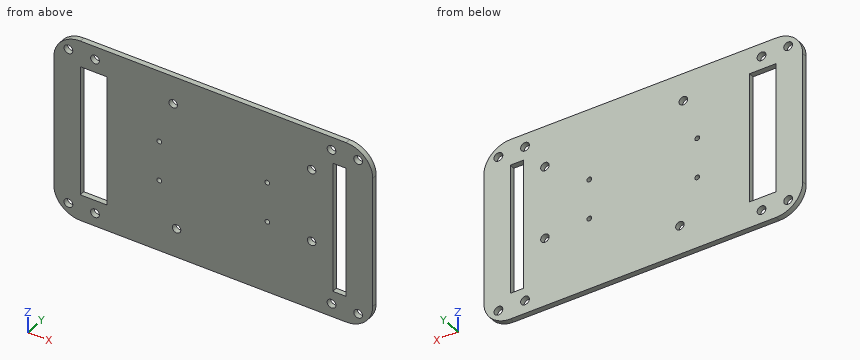
```python
from build123d import *

# Parameters (mm, degrees)
PLANTAICEZUM_W          = 120
PLANTAICEZUM_H          = 70
PLANTAICEZUM_R          = 1.6
SALIENTE_EXTRUIR3_DEPTH = 2
REDONDEO1_R             = 10
REDONDEO2_R             = 10
REDONDEO3_R             = 10
REDONDEO4_R             = 10
CROQUIS1_W              = 10
CROQUIS1_H              = 50
CROQUIS1_W_2            = 5
CORTAR_EXTRUIR1_DEPTH   = 5
CROQUIS4_R              = 1.65
CORTAR_EXTRUIR2_DEPTH   = 5
CROQUIS6_R              = 0.9
CORTAR_EXTRUIR4_DEPTH   = 10


with BuildPart() as part:
    # PlantaIceZum → Saliente-Extruir3 (new body)
    with BuildSketch(Plane(origin=(0, 0, 0), x_dir=(1, 0, 0), z_dir=(0, 1, 0))):
        with Locations((60, 35)):
            Rectangle(PLANTAICEZUM_W, PLANTAICEZUM_H)
        with Locations(Location((97, 43.66, 0), (0, 0, 270))):
            Circle(PLANTAICEZUM_R, mode=Mode.SUBTRACT)
        with Locations(Location((46.2, 58.9, 0), (0, 0, 270))):
            Circle(PLANTAICEZUM_R, mode=Mode.SUBTRACT)
        with Locations(Location((44.93, 10.64, 0), (0, 0, 270))):
            Circle(PLANTAICEZUM_R, mode=Mode.SUBTRACT)
        with Locations(Location((97, 15.72, 0), (0, 0, 270))):
            Circle(PLANTAICEZUM_R, mode=Mode.SUBTRACT)
    extrude(amount=SALIENTE_EXTRUIR3_DEPTH)

    # Redondeo1
    redondeo1_edges = [part.edges().sort_by_distance(p)[0] for p in [
        (0, 1, 0),
    ]]
    fillet(redondeo1_edges, radius=REDONDEO1_R)

    # Redondeo2
    redondeo2_edges = [part.edges().sort_by_distance(p)[0] for p in [
        (0, 1, -70),
    ]]
    fillet(redondeo2_edges, radius=REDONDEO2_R)

    # Redondeo3
    redondeo3_edges = [part.edges().sort_by_distance(p)[0] for p in [
        (120, 1, -70),
    ]]
    fillet(redondeo3_edges, radius=REDONDEO3_R)

    # Redondeo4
    redondeo4_edges = [part.edges().sort_by_distance(p)[0] for p in [
        (120, 1, 0),
    ]]
    fillet(redondeo4_edges, radius=REDONDEO4_R)

    # Croquis1 → Cortar-Extruir1 (cut)
    with BuildSketch(Plane(origin=(0, 2, 0), x_dir=(1, 0, 0), z_dir=(0, 1, 0))):
        with Locations((15, 35)):
            Rectangle(CROQUIS1_W, CROQUIS1_H)
        with Locations((107.5, 35)):
            Rectangle(CROQUIS1_W_2, CROQUIS1_H)
    extrude(amount=-CORTAR_EXTRUIR1_DEPTH, mode=Mode.SUBTRACT)

    # Croquis4 → Cortar-Extruir2 (cut)
    with BuildSketch(Plane(origin=(0, 2, 0), x_dir=(1, 0, 0), z_dir=(0, 1, 0))):
        with Locations(Location((5.5, 65, 0), (0, 0, 270))):
            Circle(CROQUIS4_R)
        with Locations(Location((114.5, 65, 0), (0, 0, 270))):
            Circle(CROQUIS4_R)
        with Locations(Location((5.5, 5, 0), (0, 0, 270))):
            Circle(CROQUIS4_R)
        with Locations(Location((114.5, 5, 0), (0, 0, 270))):
            Circle(CROQUIS4_R)
        with Locations(Location((15.5, 65, 0), (0, 0, 270))):
            Circle(CROQUIS4_R)
        with Locations(Location((104.5, 65, 0), (0, 0, 270))):
            Circle(CROQUIS4_R)
        with Locations(Location((15.5, 5, 0), (0, 0, 270))):
            Circle(CROQUIS4_R)
        with Locations(Location((104.5, 5, 0), (0, 0, 270))):
            Circle(CROQUIS4_R)
    extrude(amount=-CORTAR_EXTRUIR2_DEPTH, mode=Mode.SUBTRACT)

    # Croquis6 → Cortar-Extruir4 (cut)
    with BuildSketch(Plane(origin=(0, 2, 0), x_dir=(1, 0, 0), z_dir=(0, 1, 0))):
        with Locations(Location((39.68, 42.62, 0), (0, 0, 270))):
            Circle(CROQUIS6_R)
        with Locations(Location((39.68, 27.38, 0), (0, 0, 270))):
            Circle(CROQUIS6_R)
        with Locations(Location((80.32, 42.62, 0), (0, 0, 270))):
            Circle(CROQUIS6_R)
        with Locations(Location((80.32, 27.38, 0), (0, 0, 270))):
            Circle(CROQUIS6_R)
    extrude(amount=-CORTAR_EXTRUIR4_DEPTH, mode=Mode.SUBTRACT)


solid = part.part
```
Input: part model. Units: mm. Frame: model coordinates. Coordinates: 2 decimals unless noted, no trailing zeros. Loops run counter-clockwise (first coordinate to the right, second up) from the corner with the lowest first, then second, coordinate; pieces in that order, holes last. Notation, with made-up numbers: M 58,2.5 L 103,2.5 A36 ccw 103,37.5 Z; hole C 79.25,3.5 d6. An arc over 180 degrees is marked long. Use a Markdown table: item, result. Add a question column.
1) Line query: L1, parallel to X at y = 1.25, z = -27.38; L2, parallel to X at y = 1.5, z = -26; L3, parallel to X at y = 0.5, z = -10.64. Output: solid intervals per line, ascending. Write a range as from..to.
2) Section B-B, the plane y = 1.3. Give the number of separate pieces and of enclosed holes in the cut face, plus the area to 3 significant figures.
3) Section A-A, the plane z = -15.72. Return the cut outline in (x, y).
4) Section D-D, the plane x = 114.5. Return the cut outline in (y, z), plus the area to 3 significant figures.
5) Section C-C, the plane z = -37.5. Return the cut outline in (x, y), plus the area to 3 significant figures.
Answer below:
| question | item | result |
|---|---|---|
| 1 | L1 | 0..10, 20..38.78, 40.58..79.42, 81.22..105, 110..120 |
| 1 | L2 | 0..10, 20..105, 110..120 |
| 1 | L3 | 0..10, 20..43.33, 46.53..105, 110..120 |
| 2 | separate pieces | 1 |
| 2 | enclosed holes | 18 |
| 2 | area | 7,450 mm2 |
| 3 | outline | M 0,0 L 10,0 L 10,2 L 0,2 Z; M 20,0 L 95.4,0 L 95.4,2 L 20,2 Z; M 98.6,0 L 105,0 L 105,2 L 98.6,2 Z; M 110,0 L 120,0 L 120,2 L 110,2 Z |
| 4 | outline | M 0,-68.93 L 2,-68.93 L 2,-66.65 L 0,-66.65 Z; M 0,-63.35 L 2,-63.35 L 2,-6.65 L 0,-6.65 Z; M 0,-3.35 L 2,-3.35 L 2,-1.07 L 0,-1.07 Z |
| 4 | area | 123 mm2 |
| 5 | outline | M 0,0 L 10,0 L 10,2 L 0,2 Z; M 20,0 L 105,0 L 105,2 L 20,2 Z; M 110,0 L 120,0 L 120,2 L 110,2 Z |
| 5 | area | 210 mm2 |
